Source: CAD feature listing. Evaluate the final solid. Frame: model axes, mm. Face numbers are marked on the shaded views. A direction names the side the tool comes from. Give positions to 0.01 mm unless a question says otherwise; leave off trailing zeros. Order: outer loops, then holes, each group sorted by start corner. A loop starts at its lowest first (then second) coordinate and runs counter-clockwise, first axis right, second up. Notation, with made-up numbers: (79.25, -8.75) - (109.25, -8.75) arc R33 cw to (109.25, 22.25) - close; hole circle Ø10 at (-3.75, -39.75). An arc over 180 degrees is marked (long way). Write each question's results on one line, items separated by ' | '. Start each with the question number.
Item 1: Set-up query: the marked faces 1 and 2. Return all of +Z, -Z, +X, -X, +Y, -Y with unobstructed straight access to the full face (end or side cutting, diameter ignored); none if empty.
Item 2: Line query: line 1 along Z through (x, y) = (0, -5); line 2 along X through (y, z) = (-18.5, 0). Output: solid intervals per line, ascending.
Item 3: Contact query for flat-ended pins moving along their axis: pin 1 Ø3 at (y, z) = (-23, 4.5) entering from +X; pin 2 Ø5 at (y, z) = (-27.5, 2.5) entering from +X. Output: stop coordinate, or through.
Item 4: Section B-B on z = 4.25. Output: boundary loops of the cut face in (x, y), and give its area (3 significant figures).
Item 5: Section C-C on x = -4.75. Output: boundary loops of the cut face in (y, z), and give its area (3 significant figures).
Item 6: Section A-A on y = -14. Output: boundary loops of the cut face in (x, z), and give its area (3 significant figures).
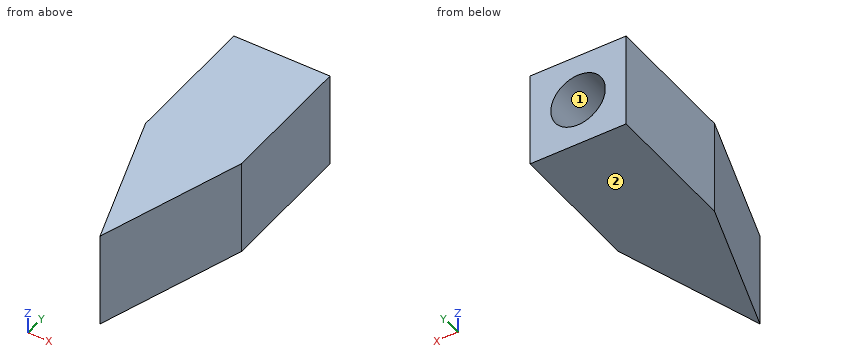
```python
from build123d import *

# Parameters (mm, degrees)
F0_W     = 12
F0_H     = 12
F1_DEPTH = 35
F3_DEPTH = 25
F5_D     = 6.8
F5_DEPTH = 22
F5_TIP   = 2.0429261047


with BuildPart() as f1:
    # F0 (on Front) → F1 (new body)
    with BuildSketch(Plane.XZ):
        Rectangle(F0_W, F0_H)
    extrude(amount=F1_DEPTH)

    # F2 (on face) → F3 (cut)
    with BuildSketch(Plane.XY.offset(6)):
        Polygon((-6, -35), (0, -35), (-6, -17), align=None)
        Polygon((6, -17), (0, -35), (6, -35), align=None)
    extrude(amount=-F3_DEPTH, mode=Mode.SUBTRACT)

    # F5
    with Locations(Plane(origin=(0, 0, 0), x_dir=(-1, 0, 0), z_dir=(0, 1, 0))):
        with Locations((0, 0)):
            Hole(F5_D / 2, depth=F5_DEPTH)
            with Locations((0, 0, -(F5_DEPTH + F5_TIP / 2))):  # 118° drill point
                Cone(0, F5_D / 2, F5_TIP, mode=Mode.SUBTRACT)


solid = f1.part
```
Evaluation:
1) face 1: +Y | face 2: -Z, +X, -X, +Y, -Y
2) line 1: z = -6 to -3.4, 3.4 to 6 | line 2: x = -5.5 to -3.4, 3.4 to 5.5
3) pin 1: stops at x = 4.5 | pin 2: stops at x = 3.33
4) outline: (-6, -17) - (0, -35) - (6, -17) - (6, 0) - (-6, 0) - close | area: 312 mm^2
5) outline: (-20.75, -6) - (0, -6) - (0, 6) - (-20.75, 6) - close | area: 249 mm^2
6) outline: (-6, -6) - (6, -6) - (6, 6) - (-6, 6) - close; hole circle Ø6.8 at (0, 0) | area: 108 mm^2
